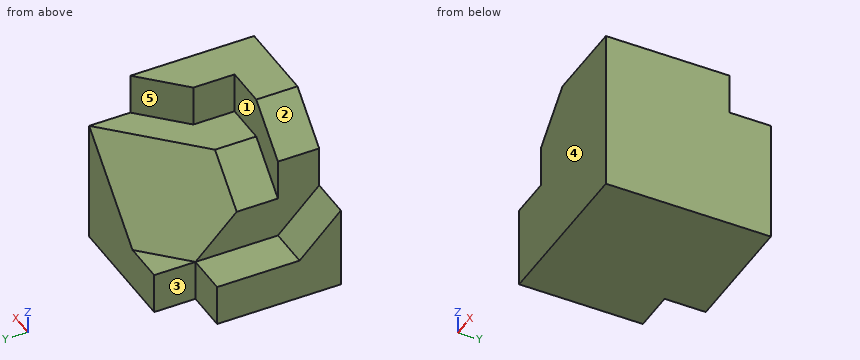
```python
from build123d import *

# Parameters (mm, degrees)
BOSS_EXTRUDE2_DEPTH = 20
BOSS_EXTRUDE4_DEPTH = 5
BOSS_EXTRUDE6_DEPTH = 20
CUT_EXTRUDE1_DEPTH  = 20
SKETCH5_W           = 5
SKETCH5_H           = 15
BOSS_EXTRUDE7_DEPTH = 5
CUT_EXTRUDE2_DEPTH  = 5
BOSS_EXTRUDE8_DEPTH = 5


with BuildPart() as part:
    # Sketch2 → Boss-Extrude2 (new body)
    with BuildSketch(Plane(origin=(0, 0, 0), x_dir=(1, 0, 0), z_dir=(0, 1, 0))):
        Polygon((-15, 0), (0, 0), (0, -15), (-10, -5), (-15, -5), align=None)
    extrude(amount=BOSS_EXTRUDE2_DEPTH)

    # Sketch3 → Boss-Extrude4 (add)
    with BuildSketch(Plane.ZY.offset(15)):
        Polygon((5, 15), (5, 5), (10, 0), (0, 0), (0, 15), align=None)
    extrude(amount=BOSS_EXTRUDE4_DEPTH)

    # Sketch4 → Boss-Extrude6 (add)
    with BuildSketch(Plane(origin=(0, 0, 0), x_dir=(-1, 0, 0), z_dir=(0, -1, 0))):
        Polygon((10, -15), (15, -10), (15, -5), (10, -5), (0, -15), align=None)
    extrude(amount=-BOSS_EXTRUDE6_DEPTH)

    # 3DSketch2 → Cut-Extrude1 (cut, along a direction that is not the sketch's normal)
    with BuildSketch(Plane(origin=(-10, 20, 5), x_dir=(0.7071067811865476, 0, 0.7071067811865475), z_dir=(0.5773502691896257, -0.577350269189626, -0.5773502691896258))):
        Polygon((0, 0), (14.142135624, 0), (7.071067812, 12.247448714), (0, 12.247448714), (-3.535533906, 6.123724357), align=None)
    extrude(amount=-CUT_EXTRUDE1_DEPTH, dir=(0, -1, 0), mode=Mode.SUBTRACT)

    # Sketch5 → Boss-Extrude7 (add)
    with BuildSketch(Plane.XY.offset(15)):
        with Locations((-2.5, 7.5)):
            Rectangle(SKETCH5_W, SKETCH5_H)
    extrude(amount=BOSS_EXTRUDE7_DEPTH)

    # Sketch6 → Cut-Extrude2 (cut)
    with BuildSketch(Plane.XY.offset(20)):
        Polygon((0, 15), (-5, 15), (-5, 10), align=None)
    extrude(amount=-CUT_EXTRUDE2_DEPTH, mode=Mode.SUBTRACT)

    # Sketch7 → Boss-Extrude8 (add)
    with BuildSketch(Plane(origin=(0, 0, 0), x_dir=(-1, 0, 0), z_dir=(0, -1, 0))):
        Polygon((15, -10), (10, -15), (5, -15), (5, -20), (10, -20), (15, -15), align=None)
    extrude(amount=-BOSS_EXTRUDE8_DEPTH)


solid = part.part
```
For this review, take the finished solid that the model builds, in its own axes (mm). Face numbers are marked on the shaded views. A direction names the side the tool comes from. Coordinates: 2 decimals unless noted, no trailing zeros. Write each loop counter-clockwise with the first axis right and the second up, starting at its lowest first coordinate (ties: lowest second). Pieces come first, ordered by that corner, then holes.
(1) The part is to be moulded in two halves that separate along X. For the marked faces 1 and 2, say which applies: +X half, -X half, draft (parallel to the pull), parting line (faces both ways), or undercut.
(2) For pin 1 Ø2.5 at (x, y) = (-12, 18.5) entering from +Z; pin 2 Ø1.5 at (y, z) = (8, 17) entering from -X; pin 3 Ø11 at (x, z) = (-11, 17.5) entering from +Y, all flat-tipped, find the tip position at first contact; note any pin that passes through.
(3) Add section D-D on x = -13.25. Give the boundary of the cut face in (y, z), then the cut area to 3 significant figures.
(4) Tool access review of the marked faces 3, 4 and 5: name each direction out of +Z, -Z, +X, -X, +Y, -Y from which nothing blocks a thin tool from reaching the whole face with its end or side.
(5) Add section A-A on x = -5.5. Give the boundary of the cut face in (y, z).
(6) Wall thickness on probe 1 along X at (y, z) = (1.75, 12.5); probe 2 along Z at (x, y) = (-1, 16.5): over which ranges is each line inside the solid? List them lowest first.
(7) Add section C-C on y = 8. Give the boundary of the cut face in (x, z), then the cut area to 4 significant figures.
(8) Add section B-B on z = 12.75. Give the boundary of the cut face in (x, y).
Answer sheet:
1. face 1: draft
1. face 2: -X half
2. pin 1: stops at z = 6.27
2. pin 2: stops at x = -5
2. pin 3: stops at y = 14.28
3. outline: (0, 0) - (20, 0) - (20, 5) - (16.75, 5) - (10, 11.75) - (5, 11.75) - (5, 16.75) - (0, 16.75) - close
3. area: 215 mm2
4. face 3: +Z, -Z, -X, +Y
4. face 4: +Z, -Z, +X, -X, -Y
4. face 5: +Z, -X, +Y
5. outline: (0, 0) - (20, 0) - (20, 9.5) - (14.5, 15) - (5, 15) - (5, 20) - (0, 20) - close
6. probe 1: x = -15 to 0
6. probe 2: z = 0 to 15
7. outline: (-20, 0) - (0, 0) - (0, 20) - (-5, 20) - (-5, 15) - (-10, 15) - (-15, 10) - (-15, 5) - (-20, 5) - close
7. area: 262.5 mm2
8. outline: (-15, 0) - (0, 0) - (0, 20) - (-2.25, 20) - (-12.25, 10) - (-12.25, 5) - (-15, 5) - close
